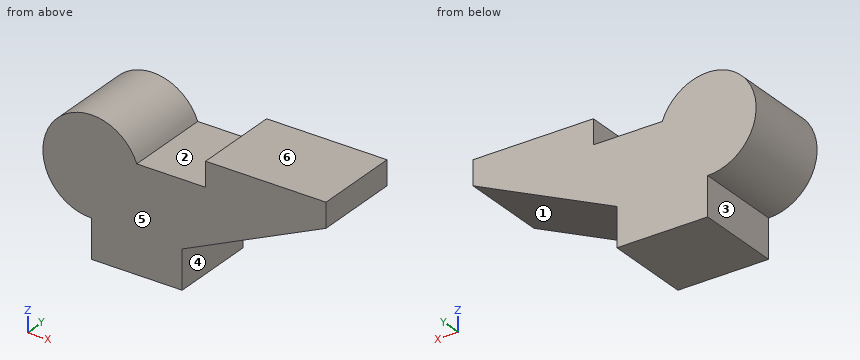
```python
from build123d import *

# Parameters (mm, degrees)
F0_W     = 79.356328
F0_H     = 33.882484
F0_W_2   = 105.214015
F0_H_2   = 21.399438
F1_DEPTH = 38.1


with BuildPart() as f1:
    # F0 (on Front) → F1 (new body, symmetric)
    with BuildSketch(Plane.XZ):
        Rectangle(F0_W, F0_H)
        with BuildLine():
            ThreePointArc((0, 74.006468), (-74.43013, 83.431692), (-39.678164, 16.941242))
            Line((-39.678164, 16.941242), (39.678164, 16.941242))
            Line((39.678164, 16.941242), (165.401873, 74.006468))
            Line((165.401873, 74.006468), (60.187858, 74.006468))
            Line((60.187858, 74.006468), (0, 74.006468))
        make_face()
        with Locations((112.794866, 84.706187)):
            Rectangle(F0_W_2, F0_H_2)
    extrude(amount=F1_DEPTH, both=True)


solid = f1.part
```
CAD build for the part. Positions are in the model's coordinates, mm. Face numbers are marked on the shaded views. A direction names the side the tool comes from. Coordinates: 2 decimals unless noted, no trailing zeros. Write each loop counter-clockwise with the first axis right and the second up, starting at its lowest first coordinate (ties: lowest second). Pieces come first, ordered by that corner, then holes. Notation, with made-up numbers: (23.25, 33) -> (52.25, 33) arc R12 ccw to (52.25, 41) -> close; hole circle Ø11 at (0, 54). An arc over 180 degrees is marked (long way). Return JSON: item names as keys, results as strings. Group by question number.
Q1. Cut at C-C, the plane z = -6.5. Give the cut face in (x, y), then the cut area to 3 significant figures.
Q2. Which spindle directions (+Z, -Z, +X, -X, +Y, -Y) get a long thin tool onto all of the face, cutting with end or side? Do the marked faces 4, 5 and 6. Say none if no direction does.
Q3. Pull direction X, two halves, no side cores. Call the marked faces 1, 2 and 3: released by +X, released by -X, zero draft, split by the parting line, or undercut.
Q4. Cut at B-B, the plane z = 88.5. Give the cut face in (x, y), then the cut area to 3 significant figures.
Q5. Flat gauge pins, fed straight in: pin 1 (23.5 mm diameter, centred on y = 10.5, z = 89, fed in from -X); pin 2 (10 mm diameter, centred on x = -46.5, y = -29, fed in from +Z); pin 3 (6 mm diameter, centred on y = 9.5, z = 32, fed in from +X). Where does each tip first touch, or does it go through?
Q6. Cut at D-D, the plane x = 28.5. Give the cut face in (y, z), then the cut area to 3 significant figures.
Q7. Cut at A-A, the plane y = 5.5. Give the cut face in (x, z), then the cut area to 3 significant figures.
Q8. Drill centre lines: line 1 (X direction, y = 18.5, z = -5); line 2 (Z direction, x = -37.5, y = 32.5); line 3 (X direction, y = 16, z = 74.5). Where is each one in solid material? Low to high.
Returned:
{
 "1": {"outline": "(-39.68, -38.1) -> (39.68, -38.1) -> (39.68, 38.1) -> (-39.68, 38.1) -> close", "area": "6,050 mm2"},
 "2": {"face 4": "-Z, +X, +Y, -Y", "face 5": "+Z, -Z, +X, -X, -Y", "face 6": "+Z, +X, +Y, -Y"},
 "3": {"face 1": "released by +X", "face 2": "undercut", "face 3": "released by -X"},
 "4": {"outline": "(-70.29, -38.1) -> (-9.07, -38.1) -> (-9.07, 38.1) -> (-70.29, 38.1) -> close; (60.19, -38.1) -> (165.4, -38.1) -> (165.4, 38.1) -> (60.19, 38.1) -> close", "area": "12,700 mm2"},
 "5": {"pin 1": "stops at x = -78", "pin 2": "stops at z = 101.56", "pin 3": "stops at x = 79.46"},
 "6": {"outline": "(-38.1, -16.94) -> (38.1, -16.94) -> (38.1, 74.01) -> (-38.1, 74.01) -> close", "area": "6,930 mm2"},
 "7": {"outline": "(-39.68, -16.94) -> (39.68, -16.94) -> (39.68, 16.94) -> (165.4, 74.01) -> (165.4, 95.41) -> (60.19, 95.41) -> (60.19, 74.01) -> (0, 74.01) arc R42.33 ccw (long way) to (-39.68, 16.94) -> close", "area": "16,700 mm2"},
 "8": {"line 1": "x = -39.68 to 39.68", "line 2": "z = -16.94 to 101.54", "line 3": "x = -79.17 to -0.19, 60.19 to 165.4"}
}
